Design review of the part built by this model. Coordinates are the model's own, in mm. Face numbers are marked on the shaded views. A direction names the side the tool comes from. Give positions to 0.01 mm unless a question says otherwise; leave off trailing zeros. Write each loop counter-clockwise with the first axis right and the second up, starting at its lowest first coordinate (ties: lowest second). Pieces come first, ordered by that corner, then holes. Notation, with made-up numbers: (-31.75, 82.25) -> (0.25, 82.25) arc R24 cw to (0.25, 98.25) -> close; hole circle Ø4 at (9, 36.25). An arc over 180 degrees is marked (long way). Write each question's results on one line, items separated by ' | '. Start each with the question number.
(1) Take a section at B-B (y = -52). State the section outline as (x, z) points.
(2) Take a section at A-A (z = 6.5). State the section outline as (x, y) points, plus the area to 3 significant figures.
(3) Clearance check with flat-ended pins moving along their axes: pin 1 (8 mm diameter, centred on x = -4, y = -11, fed in from +Z); pin 2 (1.5 mm diameter, centred on x = -2, z = 9, fed in from +Y). State where each tip first meets the part, or that it passes through.
(4) For the marked faces 1 and 2, list the 3-axis set-ups (+Z, -Z, +X, -X, +Y, -Y) from which the entire face can be reached by the end or side of a thin tool; tool diameter is ignored.
(5) To check wall thickness, follow probe 1 along X at (y, z) = (-82.2, 6.5); probe 2 along Z at (x, y) = (4, -82.2); probe 3 along Y at (x, z) = (6.25, 9). State the ranges of each line that lie inside material, in increasing order.
Autodesk Inventor part; units mm, degrees
ref_plane "YZ Plane" through (0, 0, 0) normal (1, 0, 0) x (0, 1, 0)
ref_plane "XZ Plane" through (0, 0, 0) normal (0, 1, 0) x (-1, 0, 0)
ref_plane "XY Plane" through (0, 0, 0) normal (0, 0, 1) x (1, 0, 0)
sketch "スケッチ1" plane through (0, 0, 0) normal (0, 0, 1) x (1, 0, 0)
  line L0 (-7.5, 83) -> (7.5, 83)
  line L1 (7.5, 83) -> (7.5, -83)
  line L2 (7.5, -83) -> (-7.5, -83)
  line L3 (-7.5, -83) -> (-7.5, 83)
  line L4 (-7.5, 83) -> (7.5, -83) construction
  line L5 (7.5, 83) -> (-7.5, -83) construction
  point P0 (0, 0)
  dimension "d0" = 15
  dimension "d1" = 166
extrude "押し出し1" add sketch "スケッチ1" along normal blind 1.5
sketch "スケッチ2" plane through (0, 0, 1.5) normal (0, 0, 1) x (1, 0, 0)
  line L0 (7.5, 83) -> (-7.5, 83)
  line L1 (-1.55, 3) -> (1.55, 3)
  line L2 (1.55, 3) -> (1.55, -27)
  line L3 (1.55, -27) -> (-1.55, -27)
  line L4 (-1.55, -27) -> (-1.55, 3)
  line L5 (-7.5, 83) -> (-7.5, -83)
  point P0 (0, 0)
  dimension "d6" = 3.1
  dimension "d7" = 30
  dimension "d8" = 80
  dimension "d9" = 5.95
extrude "押し出し2" cut sketch "スケッチ2" against normal blind 1.5
sketch "スケッチ3" plane through (0, 0, 1.5) normal (0, 0, 1) x (1, 0, 0)
  line L0 (-7.5, -83) -> (7.5, -83)
  line L1 (7.5, -83) -> (7.5, -81.5)
  line L2 (7.5, -81.5) -> (-7.5, -81.5)
  line L3 (-7.5, -81.5) -> (-7.5, -83)
  point P0 (0, 0)
  dimension "d12" = 1.5
extrude "押し出し3" add sketch "スケッチ3" along normal blind 10
sketch "スケッチ4" plane through (-7.5, -81.5, 1.5) normal (0, 1, 0) x (1, 0, 0)
  line L0 (15, -10) -> (0, -10)
  line L1 (15, 0) -> (15, -10)
  point P0 (7.5, 1.5)
  point P1 (11.5, -5)
  point P2 (3.5, -5)
  dimension "d15" = 8
  dimension "d16" = 5
  dimension "d17" = 3.5
hole "穴1" at (4, -81.5, 6.5) at (-4, -81.5, 6.5) direction (0, -1, 0) diameter 3.1 end through all
fillet "フィレット1" radius 4 2 edges at (-7.5, 83, 0.75) (7.5, 83, 0.75)
properties part number "pre1" material "アルミニウム 5052 H32"
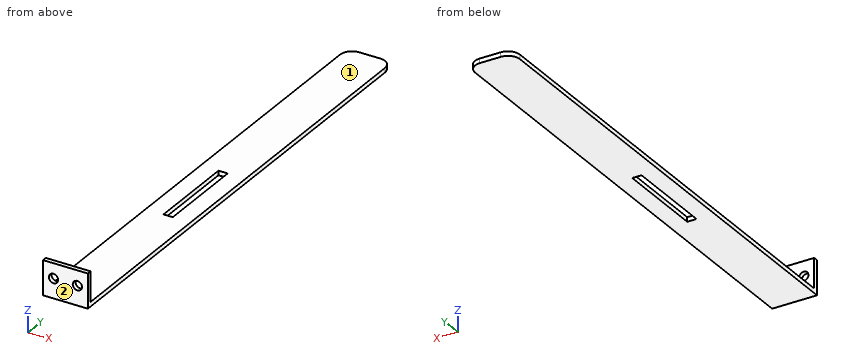
Report:
1) outline: (-7.5, 0) -> (7.5, 0) -> (7.5, 1.5) -> (-7.5, 1.5) -> close
2) outline: (-7.5, -83) -> (-5.55, -83) -> (-5.55, -81.5) -> (-7.5, -81.5) -> close; (-2.45, -83) -> (2.45, -83) -> (2.45, -81.5) -> (-2.45, -81.5) -> close; (5.55, -83) -> (7.5, -83) -> (7.5, -81.5) -> (5.55, -81.5) -> close | area: 13.2 mm2
3) pin 1: z = 1.5 | pin 2: y = -81.5
4) face 1: +Z, +X, -X, +Y | face 2: +Z, -Z, +X, -X, -Y
5) probe 1: -7.5 to -5.55, -2.45 to 2.45, 5.55 to 7.5 | probe 2: 0 to 4.95, 8.05 to 11.5 | probe 3: -83 to -81.5
